Source: CAD feature listing. Evaluate the final solid. Frame: model axes, mm. Face numbers are marked on the shaded views. A direction names the side the tool comes from. Give positions to 0.01 mm unless a question says otherwise; leave off trailing zeros. Write each loop counter-clockwise with the first axis right and the second up, starting at its lowest first coordinate (ties: lowest second). Pieces come first, ordered by that corner, then holes. Notation, with made-up numbers: (37.25, 67) -> (94.25, 67) arc R12 ccw to (94.25, 80) -> close; hole circle Ø11 at (37.5, 3). An arc over 180 degrees is marked (long way). Write item = value, one per line.
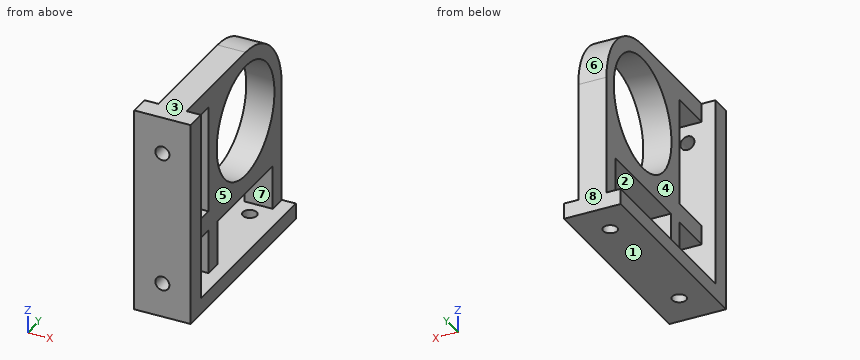
from build123d import *

# Parameters (mm, degrees)
SKETCH1_R                = 25.4635
BOSS_EXTRUDE1_DEPTH      = 12.7
BOSS_EXTRUDE2_DEPTH      = 6.35
BOSS_EXTRUDE2_DEPTH_BACK = 19.05
SKETCH4_W                = 20.078494948
SKETCH4_H                = 48.78095735
SKETCH4_W_2              = 48.420880553
SKETCH4_H_2              = 19.195923741
CUT_EXTRUDE2_DEPTH       = 26.162
SKETCH5_R                = 3.175
CUT_EXTRUDE3_DEPTH       = 11.43
SKETCH6_R                = 3.175
CUT_EXTRUDE4_DEPTH       = 11.43


with BuildPart() as part:
    # Sketch1 → Boss-Extrude1 (new body)
    with BuildSketch(Plane(origin=(0, 0, 0), x_dir=(0, 0, -1), z_dir=(1, 0, 0))):
        with BuildLine():
            Line((0, 31.882172919), (31.882172919, 31.882172919))
            Line((31.882172919, 31.882172919), (60.87463474, 31.882172919))
            Line((60.87463474, 31.882172919), (60.87463474, -60.96))
            Line((60.87463474, -60.96), (-31.882172919, -60.96))
            Line((-31.882172919, -60.96), (-31.882172919, 0))
            ThreePointArc((-31.882172919, 0), (-22.54410067, 22.54410067), (0, 31.882172919))
        make_face()
        Circle(SKETCH1_R, mode=Mode.SUBTRACT)
    extrude(amount=BOSS_EXTRUDE1_DEPTH)

    # Sketch8 → Boss-Extrude2 (add, two sides: drawn at the far end of the back side and taken through both)
    with BuildSketch(Plane(origin=(12.7, 0, 0), x_dir=(0, 0, -1), z_dir=(1, 0, 0)).offset(-BOSS_EXTRUDE2_DEPTH_BACK)):
        Polygon((60.87463474, 31.882172919), (53.770648903, 31.882172919), (53.770648903, -51.937867719), (-31.882172919, -51.937867719), (-31.882172919, -60.96), (53.770648903, -60.96), (60.87463474, -60.96), align=None)
    extrude(amount=BOSS_EXTRUDE2_DEPTH + BOSS_EXTRUDE2_DEPTH_BACK)

    # Sketch4 → Cut-Extrude2 (cut)
    with BuildSketch(Plane.ZY):
        with Locations((-43.731401429, -0.427222634)):
            Rectangle(SKETCH4_W, SKETCH4_H)
        with Locations((-0.75610861, -42.339905849)):
            Rectangle(SKETCH4_W_2, SKETCH4_H_2)
        with Locations((-43.731401429, -42.339905849)):
            Rectangle(SKETCH4_W, SKETCH4_H_2)
    extrude(amount=-CUT_EXTRUDE2_DEPTH, mode=Mode.SUBTRACT)

    # Sketch5 → Cut-Extrude3 (cut)
    with BuildSketch(Plane(origin=(0, 0, -60.87463474), x_dir=(-1, 0, 0), z_dir=(0, 0, -1))):
        with Locations((-6.35, 16.187024645)):
            Circle(SKETCH5_R)
        with Locations((-6.35, -44.788648077)):
            Circle(SKETCH5_R)
    extrude(amount=-CUT_EXTRUDE3_DEPTH, mode=Mode.SUBTRACT)

    # Sketch6 → Cut-Extrude4 (cut)
    with BuildSketch(Plane.XZ.offset(60.96)):
        with Locations(Location((6.35, 15.24, 0), (0, 0, 270))):
            Circle(SKETCH6_R)
        with Locations(Location((6.35, -45.41055385, 0), (0, 0, 270))):
            Circle(SKETCH6_R)
    extrude(amount=-CUT_EXTRUDE4_DEPTH, mode=Mode.SUBTRACT)


solid = part.part
1) Cut plane C-C (z = 15.24). Return the cut outline in (x, y) (3 decimals).
Computed:
outline = (-6.35, -60.96) -> (3.175, -60.96) -> (3.175, -51.938) -> (-6.35, -51.938) -> close; (0, -32.742) -> (12.7, -32.742) -> (12.7, -20.399) -> (0, -20.399) -> close; (0, 20.399) -> (12.7, 20.399) -> (12.7, 28.004) -> (0, 28.004) -> close; (9.525, -60.96) -> (19.05, -60.96) -> (19.05, -51.938) -> (9.525, -51.938) -> close
2) Material intervals for L1, parallel to Y at x = 6.35, z = -55.25; L2, parallel to Y at x = 2, z = -45; L3, parallel to Z at x = 8.25, y = -40.5, sorted ascending.
Computed:
L1 = -60.96 to -47.96, -41.61 to 13.01, 19.36 to 31.88
L2 = -60.96 to -51.94, -32.74 to -24.82, 23.96 to 31.88
L3 = -60.87 to -53.77, -33.69 to -24.97, 23.45 to 31.88
3) Cut plane B-B (x = 11.5). Return the cut outline in (y, z).
Computed:
outline = (-60.96, -60.87) -> (31.88, -60.87) -> (31.88, 0) arc R31.88 ccw to (0, 31.88) -> (-60.96, 31.88) -> close; hole (-51.94, -53.77) -> (-32.74, -53.77) -> (-32.74, -33.69) -> (-51.94, -33.69) -> close; hole (-51.94, -24.97) -> (-32.74, -24.97) -> (-32.74, 23.45) -> (-51.94, 23.45) -> close; hole circle Ø50.93 at (0, 0); hole (-24.82, -53.77) -> (23.96, -53.77) -> (23.96, -33.69) -> (-24.82, -33.69) -> close
4) Contact query for flat-ended pins moving along their axis: pin 1 (12 mm diameter, centred on y = -8, z = -35.5, fed in from +X); pin 2 (10 mm diameter, centred on x = 6.35, y = 16.19, fed in from +Z); pin 3 (5 mm diameter, centred on x = 6.35, y = -44.79, fed in from -Z). Output: stop coordinate, or through.
Computed:
pin_1 = 12.7
pin_2 = 29.85
pin_3 = -33.69
5) Cut plane A-A (x = 6.35). State how many separate pieces and enclosed holes the cut face has, then the cut area to 3 significant figures.
Computed:
separate_pieces = 2
enclosed_holes = 1
area = 3,860 mm²
6) Cut plane D-D (x = 17). Return the cut outline in (y, z), then the cut area to 3 significant figures.
Computed:
outline = (-60.96, -60.87) -> (31.88, -60.87) -> (31.88, -53.77) -> (-51.94, -53.77) -> (-51.94, 31.88) -> (-60.96, 31.88) -> close
area = 1,430 mm²
7) Draft query along Z for the marked faces 6, 7 and 8. Return one class per face: pulls with the +Z half, pulls with the -Z half, needs draft (parallel to the pull), parting line crosses it, or undercut.
Computed:
face_6 = pulls with the +Z half
face_7 = undercut
face_8 = needs draft
8) Access query for the marked faces 1, 2, 3, 4 and 5. Directions: +Z, -Z, +X, -X, +Y, -Y. A direction counts if a zero-diameter tool reaches every point of the face in a straight line with its end or side. Return the directions, or none.
Computed:
face_1 = -Z, +X, -X, +Y, -Y
face_2 = +X, -X
face_3 = +Z, +X, -X, +Y, -Y
face_4 = +Z, -X, +Y
face_5 = +Z, +X, +Y
